Source: CAD feature listing. Evaluate the final solid. Frame: model axes, mm. A direction names the side the tool comes from. Give positions to 0.01 mm unless a question says otherwise; leave off trailing zeros. Write each loop counter-clockwise with the first axis right and the second up, starting at its lowest first coordinate (ties: lowest second). Pieces come first, ordered by that corner, then holes. Notation, with made-up numbers: (47, 15.25) -> (84, 15.25) arc R18 ccw to (84, 47.25) -> close; hole circle Ø2 at (-1.75, -28). An arc over 180 degrees is marked (long way). Answer as a JSON object with one key per item and string values. Group by question number.
Item 1: Access query for faces 5 (the face through (81.133, 60.534, 1.479)), 6 (the face through (78.963, 35, 1)). Directions: +Z, -Z, +X, -X, +Y, -Y. A direction counts if a zero-diameter tool reaches every point of the face in a straight line with its end or side. Return the directions, or none.
Item 2: First-contact query: pin 1 Ø1.5 at (y, z) = (43.5, 1) entering from +X; pin 2 Ø0.9 at (x, z) = (43.5, 2) entering from +Y. Flat tips, straight axial feed; report the tip coordinate or a pass-through.
Item 3: Section query B-B on x = 70. Return the cut outline in (y, z), plus the area to 3 significant figures.
Item 4: Pull-direction query (X, two-part tool) for faces 1 (the face through (29.463, 21, 1)), 2 (the face through (74.463, 21, 1)), 3 (the face through (55.14, 65.95, 1.48)), 4 (the face through (52, 11.796, 1)); classes: pulls with the +X half, pulls with the -X half, needs draft (parallel to the pull), parting line crosses it, or undercut.
Item 5: Section query D-D on z = 2.3. Give the number of separate pieces and of enclosed holes in the cut face, plus the area to 3 significant figures.
Item 6: Section query C-C on x = 51.5. Return the cut outline in (y, z).
Item 7: Ray query, probe 1 along X at (y, z) = (49, 2.75); probe 2 along Y at (x, z) = (78.5, 1); probe 3 along Y at (x, z) = (66, 2.6). Return the intervals inside material, ascending. Write a range as from..to.
Item 8: Section query A-A on x = 41. Return the cut outline in (y, z), plus the area to 3 significant figures.
from build123d import *

# Parameters (mm, degrees)
MODEL_R             = 1.3
MODEL_R_2           = 1.500000002
MODEL_W             = 3
MODEL_H             = 10
MODEL_W_2           = 10
MODEL_H_2           = 3
MODEL_H_3           = 6
MODEL_W_3           = 22.8
MODEL_H_4           = 12.2
BOSS_EXTRUDE1_DEPTH = 3


with BuildPart() as part:
    # Model → Boss-Extrude1 (new body)
    with BuildSketch(Plane.XY):
        with BuildLine():
            Line((21.96271471, 39.580829954), (21.96276757, 58.495922142))
            ThreePointArc((21.96276757, 58.495922142), (22.066046655, 59.276171923), (22.368675297, 60.00272006))
            Line((22.368675297, 60.00272006), (25.427717727, 65.269480806))
            Line((25.427717727, 65.269480806), (27.25161841, 68.40969502))
            ThreePointArc((27.25161841, 68.40969502), (29.03985645, 70.035063012), (31.437828278, 70.333973552))
            Line((31.437828278, 70.333973552), (79.508282697, 61.445627037))
            ThreePointArc((79.508282697, 61.445627037), (81.151311996, 60.514547069), (81.963503617, 58.809613066))
            Line((81.963503617, 58.809613066), (81.989341148, 57.295464993))
            Line((81.989341148, 57.295464993), (81.962758854, 14.795654622))
            ThreePointArc((81.962758854, 14.795654622), (81.08382665, 12.674474539), (78.962495601, 11.795906758))
            Line((78.962495601, 11.795906758), (24.962535775, 11.795906758))
            ThreePointArc((24.962535775, 11.795906758), (22.841288266, 12.674619651), (21.962651159, 14.795898552))
            Line((21.962651159, 14.795898552), (21.96271471, 39.580829954))
        make_face()
        with Locations((61.462672705, 58.495778552)):
            Circle(MODEL_R, mode=Mode.SUBTRACT)
        with Locations((61.462672705, 40.495778552)):
            Circle(MODEL_R, mode=Mode.SUBTRACT)
        with Locations((30.710508107, 66.400677282)):
            Circle(MODEL_R, mode=Mode.SUBTRACT)
        with Locations((51.962675263, 20.995768297)):
            Circle(MODEL_R_2, mode=Mode.SUBTRACT)
        with Locations((77.462616288, 28.995637525)):
            Circle(MODEL_R_2, mode=Mode.SUBTRACT)
        with Locations((30.962567569, 46.495883681)):
            Rectangle(MODEL_W, MODEL_H, mode=Mode.SUBTRACT)
        with Locations((34.462567569, 20.995883681)):
            Rectangle(MODEL_W_2, MODEL_H_2, mode=Mode.SUBTRACT)
        with Locations((69.462567569, 20.995883681)):
            Rectangle(MODEL_W_2, MODEL_H_2, mode=Mode.SUBTRACT)
        with Locations((77.462598338, 22.495645219)):
            Rectangle(MODEL_W, MODEL_H_3, mode=Mode.SUBTRACT)
        with Locations((61.462721415, 49.495778552)):
            Rectangle(MODEL_W_3, MODEL_H_4, mode=Mode.SUBTRACT)
        with Locations((77.462598338, 35.495645219)):
            Rectangle(MODEL_W, MODEL_H_3, mode=Mode.SUBTRACT)
        with Locations((44.462670134, 27.495883681)):
            Rectangle(MODEL_W_2, MODEL_H_3, mode=Mode.SUBTRACT)
    extrude(amount=BOSS_EXTRUDE1_DEPTH)


solid = part.part
Worked answers:
{
 "1": {"face 5": "+Z, -Z, +X, +Y", "face 6": "+Z, -Z"},
 "2": {"pin 1": "x = 81.98", "pin 2": "y = 68.19"},
 "3": {"outline": "(11.8, 0) -> (19.5, 0) -> (19.5, 3) -> (11.8, 3) -> close; (22.5, 0) -> (43.4, 0) -> (43.4, 3) -> (22.5, 3) -> close; (55.6, 0) -> (63.2, 0) -> (63.2, 3) -> (55.6, 3) -> close", "area": "109 mm^2"},
 "4": {"face 1": "undercut", "face 2": "undercut", "face 3": "pulls with the +X half", "face 4": "needs draft"},
 "5": {"separate pieces": "1", "enclosed holes": "12", "area": "2,740 mm^2"},
 "6": {"outline": "(11.8, 0) -> (19.57, 0) -> (19.57, 3) -> (11.8, 3) -> close; (22.42, 0) -> (43.4, 0) -> (43.4, 3) -> (22.42, 3) -> close; (55.6, 0) -> (66.62, 0) -> (66.62, 3) -> (55.6, 3) -> close"},
 "7": {"probe 1": "21.96..29.46, 32.46..50.06, 72.86..81.98", "probe 2": "11.8..19.5, 25.5..27.91, 30.08..32.5, 38.5..61.63", "probe 3": "11.8..19.5, 22.5..43.4, 55.6..63.94"},
 "8": {"outline": "(11.8, 0) -> (24.5, 0) -> (24.5, 3) -> (11.8, 3) -> close; (30.5, 0) -> (68.57, 0) -> (68.57, 3) -> (30.5, 3) -> close", "area": "152 mm^2"}
}
